from build123d import *

# Parameters (mm, degrees)
SKETCH1_W           = 53
SKETCH1_H           = 36
BOSS_EXTRUDE1_DEPTH = 13
CUT_EXTRUDE1_DEPTH  = 54


with BuildPart() as part:
    # Sketch1 → Boss-Extrude1 (new body)
    with BuildSketch(Plane(origin=(0, 0, 0), x_dir=(1, 0, 0), z_dir=(0, 1, 0))):
        Rectangle(SKETCH1_W, SKETCH1_H)
    extrude(amount=BOSS_EXTRUDE1_DEPTH)

    # Sketch2 → Cut-Extrude1 (cut, through all)
    with BuildSketch(Plane(origin=(26.5, 0, 0), x_dir=(0, 0, -1), z_dir=(1, 0, 0))):
        with BuildLine():
            Line((-18, 13), (-15, 13))
            ThreePointArc((-15, 13), (-17.121320344, 12.121320344), (-18, 10))
            Line((-18, 10), (-18, 13))
        make_face()
        with BuildLine():
            Line((15, 13), (18, 13))
            Line((18, 13), (18, 10))
            ThreePointArc((18, 10), (17.121320344, 12.121320344), (15, 13))
        make_face()
    extrude(amount=-CUT_EXTRUDE1_DEPTH, mode=Mode.SUBTRACT)


solid = part.part
Can you work these out from the model? Positions are in its coordinate system, mm. Coordinates: 2 decimals unless noted, no trailing zeros. Write each loop counter-clockwise with the first axis right and the second up, starting at its lowest first coordinate (ties: lowest second). Pieces come first, ordered by that corner, then holes.
Q1. Imagine slicing it at A-A, the plane z = 16.5. List the corners of the cut face in (x, y) for me, plus the area to 3 significant figures.
Results found:
outline: (-26.5, 0) - (26.5, 0) - (26.5, 12.6) - (-26.5, 12.6) - close
area: 668 mm2
Q2. Please list where these lines run through material, in increasing order: L1, parallel to Y at x = -10, z = 16; L2, parallel to Z at x = -2, y = 12; L3, parallel to Z at x = -2.5, y = 11.75.
Results found:
L1: y = 0 to 12.83
L2: z = -17.24 to 17.24
L3: z = -17.44 to 17.44
Q3. Imagine slicing it at B-B, the plane y = 12.25. List the corners of the cut face in (x, z) for me, plus the area to 3 significant figures.
Results found:
outline: (-26.5, -16.98) - (26.5, -16.98) - (26.5, 16.98) - (-26.5, 16.98) - close
area: 1,800 mm2
